from build123d import *

# Parameters (mm, degrees)
F0_W     = 40
F0_H     = 50
F1_DEPTH = 60
F2_W     = 40
F2_H     = 20
F3_DEPTH = 30
F5_DEPTH = 60.001
F6_W     = 10
F6_H     = 10
F7_DEPTH = 40.001
F8_R     = 20


with BuildPart() as f1:
    # F0 (on Right) → F1 (new body)
    with BuildSketch(Plane.YZ):
        with Locations((20, 25)):
            Rectangle(F0_W, F0_H)
    extrude(amount=F1_DEPTH)

    # F2 (on face) → F3 (cut)
    with BuildSketch(Plane.YZ.offset(60)):
        with Locations((20, 40)):
            Rectangle(F2_W, F2_H)
    extrude(amount=-F3_DEPTH, mode=Mode.SUBTRACT)

    # F4 (on face) → F5 (cut, through all)
    with BuildSketch(Plane.YZ.offset(60)):
        with BuildLine():
            ThreePointArc((10, 30), (20, 20), (30, 30))
            Line((30, 30), (10, 30))
        make_face()
        with BuildLine():
            Line((10, 30), (30, 30))
            ThreePointArc((30, 30), (20, 40), (10, 30))
        make_face()
    extrude(amount=-F5_DEPTH, mode=Mode.SUBTRACT)

    # F6 (on face) → F7 (cut, through all)
    with BuildSketch(Plane.XZ):
        with Locations((55, 5)):
            Rectangle(F6_W, F6_H)
    extrude(amount=-F7_DEPTH, mode=Mode.SUBTRACT)

    # F8
    f8_edges = [f1.edges().sort_by_distance(p)[0] for p in [
        (15, 0, 50),
    ]]
    fillet(f8_edges, radius=F8_R)


solid = f1.part
Here's how the part is built. I have some questions about the finished solid (model axes, mm). A direction names the side the tool comes from. Round coordinates to 2 decimals unless told otherwise and drop trailing zeros. Loops run counter-clockwise (first coordinate to the right, second up) from the corner with the lowest first, then second, coordinate; pieces in that order, holes last. Notation, with made-up numbers: (63.5, 73.5) - (104.5, 73.5) arc R16 ccw to (104.5, 94.5) - close; hole circle Ø9 at (60.25, -36). An arc over 180 degrees is marked (long way). One line per question, with ' | ' between items. Start each with the question number.
Q1. I want a section at D-D (x = 46.5). Write out the boundary of the cut face in (y, z), then the cut area to 3 significant figures.
Q2. I want a section at C-C (z = 25.5). Write out the boundary of the cut face in (x, y).
Q3. I want a section at B-B (y = 13.5). Write out the boundary of the cut face in (x, z), then the cut area to 3 significant figures.
Q4. We'd pull the mould along Y, two halves only. Please class faces 4 (the cylindrical face through (23.75, 17.83, 20.24)), 5 (the flat face through (30, 24, 40)), 6 (the flat face through (23, 40, 19)): +Y half, -Y half, draft (parallel to the pull), parting line (faces both ways), or undercut.
Q5. For faces 1 (the flat face through (60, 20, 18)), 2 (the flat face through (45, 35, 30)), 3 (the flat face through (55, 20, 10)), which set-ups out of +Z, -Z, +X, -X, +Y, -Y let a thin tool reach every point of the face, with its end or its side?
Q6. Please list where these lines run through material, in increasing order: line 1 (X direction, y = 5, z = 41.5); line 2 (Y direction, x = 12.5, z = 29.5); line 3 (Z direction, x = 10, y = 14). Write a range as [from, to].
Q7. I want a section at A-A (x = 14). Write out the boundary of the cut face in (y, z), then the cut area to 3 significant figures.
Q8. Will these pins go through, and if not, where does the flat tip stop? pin 1 (2 mm diameter, centred on x = 40, y = 17.5, fed in from +Z); pin 2 (4 mm diameter, centred on y = 20, z = 43.5, fed in from +X); pin 3 (2 mm diameter, centred on x = 25, z = 35.5, fed in from -Y).
Response values:
1) outline: (0, 0) - (40, 0) - (40, 30) - (30, 30) arc R10 cw to (10, 30) - (0, 30) - close | area: 1,040 mm²
2) outline: (0, 0) - (60, 0) - (60, 11.07) - (0, 11.07) - close; (0, 28.93) - (60, 28.93) - (60, 40) - (0, 40) - close
3) outline: (0, 0) - (50, 0) - (50, 10) - (60, 10) - (60, 22.4) - (0, 22.4) - close; (0, 37.6) - (30, 37.6) - (30, 48.91) - (0, 48.91) - close | area: 1,580 mm²
4) face 4: undercut | face 5: draft | face 6: +Y half
5) face 1: +Z, -Z, +X, +Y, -Y | face 2: +Z, +X, +Y, -Y | face 3: -Z, +X, +Y, -Y
6) line 1: x = [0, 30] | line 2: y = [0, 10.01], [29.99, 40] | line 3: z = [0, 22], [38, 49.08]
7) outline: (0, 0) - (40, 0) - (40, 50) - (20, 50) arc R20 ccw to (0, 30) - close; hole circle Ø20 at (20, 30) | area: 1,600 mm²
8) pin 1: stops at z = 20.63 | pin 2: stops at x = 30 | pin 3: stops at y = 0.51
